```python
from build123d import *

# Parameters (mm, degrees)
SKETCH_W      = 100
SKETCH_H      = 85
PAD_DEPTH     = 5
SKETCH001_W   = 55
SKETCH001_H   = 28
SKETCH001_W_2 = 25
SKETCH001_H_2 = 55
SKETCH001_W_3 = 20
SKETCH001_H_3 = 20
PAD001_DEPTH  = 16
SKETCH002_W   = 35
SKETCH002_H   = 20
SKETCH002_W_2 = 10
PAD002_DEPTH  = 11.5


with BuildPart() as pad002:
    # Sketch → Pad (new body)
    with BuildSketch(Plane.XY):
        with Locations((50, -42.5)):
            Rectangle(SKETCH_W, SKETCH_H)
    extrude(amount=-PAD_DEPTH)

    # Sketch001 → Pad001 (new body)
    with BuildSketch(Plane.XY):
        with Locations((27.5, -14)):
            Rectangle(SKETCH001_W, SKETCH001_H)
        with BuildLine():
            ThreePointArc((13.492439, -5.458467), (4.492439, -14.458467), (13.492439, -23.458467))
            Line((13.492439, -23.458467), (41.492439, -23.458467))
            ThreePointArc((41.492439, -23.458467), (50.492439, -14.458467), (41.492439, -5.458467))
            Line((13.492439, -5.458467), (41.492439, -5.458467))
        make_face(mode=Mode.SUBTRACT)
        with Locations((87.5, -42.5)):
            Rectangle(SKETCH001_W_2, SKETCH001_H_2)
        with BuildLine():
            ThreePointArc((96.279266, -26.175545), (87.343376, -17.239655), (78.407486, -26.175545))
            Line((78.407486, -26.175545), (78.407486, -58.197685))
            ThreePointArc((78.407486, -58.197685), (87.343376, -67.133575), (96.279266, -58.197685))
            Line((96.279266, -26.175545), (96.279266, -58.197685))
        make_face(mode=Mode.SUBTRACT)
        with Locations((10, -55)):
            Rectangle(SKETCH001_W_3, SKETCH001_H_3)
    extrude(amount=PAD001_DEPTH)

    # Sketch002 → Pad002 (new body)
    with BuildSketch(Plane.XY):
        with Locations((17.5, -75)):
            Rectangle(SKETCH002_W, SKETCH002_H)
        with Locations((31, -38)):
            Rectangle(SKETCH002_W_2, SKETCH002_H)
    extrude(amount=PAD002_DEPTH)


with BuildPart() as part_mirroring:
    # Part__Mirroring: instance of Pad002
    add(pad002.part.mirror(Plane(origin=(0, 0, 0), x_dir=(0, 1, 0), z_dir=(0, 0, 1))))


solid = part_mirroring.part
```
Here's how the part is built. I have some questions about the finished solid (model axes, mm). A direction names the side the tool comes from. Give positions to 0.01 mm unless a question says otherwise; leave off trailing zeros. Loops run counter-clockwise (first coordinate to the right, second up) from the corner with the lowest first, then second, coordinate; pieces in that order, holes last. Notation, with made-up numbers: M 26.5,45 L 36.5,45 A11 cw 36.5,56 Z; hole C 66,-6 d5. An arc over 180 degrees is marked long. Put each result on its own line as item: value. Start each with the question number.
(1) I want a section at C-C on x = 28. Please give me the cut outline in (y, z), then the cut area to 4 significant figures.
(2) I need wall thicknesses on line 1 along Y through (x, z) = (15.5, -2.75); line 2 along X through (y, z) = (-46.5, -10); line 3 along X through (y, z) = (-28.5, -1.75). Which ranges of each line are inside material? Lowest first, please. Write a range as [from, to].
(3) I want a section at D-D on x = 38.5. Please give me the cut outline in (y, z).
(4) For faces 1 (the flat face through (27, -28, -13)), 2 (the flat face through (36, -38, -6)), 3 (the flat face through (75, -43, -8)), 4 (the flat face through (17, -75, -11.5)), which set-ups out of +Z, -Z, +X, -X, +Y, -Y let a thin tool reach every point of the face, with its end or its side?
(5) I want a section at A-A on z = -4.5. Please give me the cut outline in (x, y).
(6) If we mould it in two halves opening along Y, with no side actions, what happens to faces 5 (the flat face through (87, -70, -8)), 6 (the flat face through (87, -15, -8)), 7 (the flat face through (10, -55, -16)), 8 (the flat face through (10, -45, -8))? For each: +Y half, -Y half, draft (parallel to the pull), parting line (faces both ways), or undercut.
(7) I want a section at B-B on y = -31.5. Please give me the cut outline in (x, z).
(8) Will these pins go through, and if not, where does the flat tip stop? pin 1 Ø8 at (y, z) = (-18, -12.5) entering from -X; pin 2 Ø8 at (y, z) = (-37.5, -13) entering from -X; pin 3 Ø3 at (x, y) = (32.5, -37.5) entering from -Z; pin 4 Ø2 at (x, z) = (6, -13.5) entering from -Y.
Answer block:
1. outline: M -85,-11.5 L -65,-11.5 L -65,0 L -48,0 L -48,-11.5 L -28,-11.5 L -28,-16 L -23.46,-16 L -23.46,0 L -5.46,0 L -5.46,-16 L 0,-16 L 0,5 L -85,5 Z
1. area: 1,045 mm^2
2. line 1: [-85, -45], [-28, -23.46], [-5.46, 0]
2. line 2: [0, 20], [26, 36], [75, 78.41], [96.28, 100]
2. line 3: [26, 36], [75, 78.41], [96.28, 100]
3. outline: M -85,0 L -28,0 L -28,-16 L -23.46,-16 L -23.46,0 L -5.46,0 L -5.46,-16 L 0,-16 L 0,5 L -85,5 Z
4. face 1: -Z
4. face 2: -Z, -Y
4. face 3: -Z, +Y, -Y
4. face 4: -Z, -X, -Y
5. outline: M 0,-85 L 35,-85 L 35,-65 L 20,-65 L 20,-45 L 0,-45 Z; M 0,-28 L 26,-28 L 26,-48 L 36,-48 L 36,-28 L 55,-28 L 55,0 L 0,0 Z; M 75,-70 L 100,-70 L 100,-15 L 75,-15 Z; hole M 13.49,-23.46 L 41.49,-23.46 A9 ccw 41.49,-5.46 L 13.49,-5.46 A9 ccw Z; hole M 78.41,-58.2 A8.94 ccw 96.28,-58.2 L 96.28,-26.18 A8.94 ccw 78.41,-26.18 Z
6. face 5: -Y half
6. face 6: +Y half
6. face 7: draft
6. face 8: undercut
7. outline: M 0,0 L 26,0 L 26,-11.5 L 36,-11.5 L 36,0 L 75,0 L 75,-16 L 78.41,-16 L 78.41,0 L 96.28,0 L 96.28,-16 L 100,-16 L 100,5 L 0,5 Z
8. pin 1: x = 0
8. pin 2: x = 26
8. pin 3: z = -11.5
8. pin 4: y = -65
